CAD build for the part. Positions are in the model's coordinates, mm. A direction names the side the tool comes from. Coordinates: 2 decimals unless noted, no trailing zeros. Write item = value, one per line. Start each with the question number.
```python
from build123d import *

# Parameters (mm, degrees)
SKETCH1_R           = 10.9
BOSS_EXTRUDE1_DEPTH = 10
FILLET5_R           = 1
FILLET1_R           = 1
SKETCH3_R           = 2
CUT_EXTRUDE2_DEPTH  = 8
SKETCH6_R           = 11.874719229
SKETCH6_R_2         = 5
BOSS_EXTRUDE3_DEPTH = 3


with BuildPart() as part:
    # Sketch1 → Boss-Extrude1 (new body)
    with BuildSketch(Plane.XY):
        with BuildLine():
            Line((18.000000111, 2.53629242), (18.000000111, -9))
            Line((18.000000111, -9), (-17.965840671, -9))
            Line((-17.965840671, -9), (-17.965840671, 23.5))
            ThreePointArc((-17.965840671, 23.5), (-0.099999918, 41.365840754), (17.765840836, 23.5))
            Line((17.765840836, 23.5), (18.000000111, 16.187309001))
            Line((18.000000111, 16.187309001), (18.000000111, 14.96196947))
            Line((18.000000111, 14.96196947), (18.000000111, 2.53629242))
        make_face()
        with Locations((-0.099999918, 23.5)):
            Circle(SKETCH1_R, mode=Mode.SUBTRACT)
        with BuildLine():
            Line((-4.4, 1), (-5.2, 1))
            Line((-5.2, 1), (-6, 0.2))
            Line((-6, 0.2), (-6, -3.6))
            ThreePointArc((-6, -3.6), (-5.882842712, -3.882842712), (-5.6, -4))
            Line((-5.6, -4), (5.6, -4))
            ThreePointArc((5.6, -4), (5.882842712, -3.882842712), (6, -3.6))
            Line((6, -3.6), (6, 0.2))
            Line((6, 0.2), (5.2, 1))
            Line((5.2, 1), (4.4, 1))
            Line((4.4, 1), (4.4, 2))
            Line((4.4, 2), (5.2, 2))
            Line((5.2, 2), (6, 2.8))
            Line((6, 2.8), (6, 3.6))
            ThreePointArc((6, 3.6), (5.882842712, 3.882842712), (5.6, 4))
            Line((5.6, 4), (-5.6, 4))
            ThreePointArc((-5.6, 4), (-5.882842712, 3.882842712), (-6, 3.6))
            Line((-6, 3.6), (-6, 2.8))
            Line((-6, 2.8), (-5.2, 2))
            Line((-5.2, 2), (-4.4, 2))
            Line((-4.4, 2), (-4.4, 1))
        make_face(mode=Mode.SUBTRACT)
    extrude(amount=-BOSS_EXTRUDE1_DEPTH)

    # Fillet5
    fillet5_edges = [part.edges().sort_by_distance(p)[0] for p in [
        (18.000000111, -9, -5),
        (-17.965840671, -9, -5),
        (0.01707972, -9, -10),
        (0.01707972, -9, 0),
    ]]
    fillet(fillet5_edges, radius=FILLET5_R)

    # Fillet1
    # the kernel refuses this fillet: 1 mm, written as the material it adds along each edge
    with BuildSketch(Plane(origin=(17.765840836, 23.5, 0), x_dir=(0.032004541259538756, -0.9994877234557543, 0), z_dir=(0, 0, -1))) as fillet1_piece_1:
        with BuildLine():
            CenterArc((0.015788393, -1), FILLET1_R, 90, 1.784765128)
            ThreePointArc((-0.015356597, -0.000485123), (-0.007678246, -0.000244212), (0, 0))
            Line((0, 0), (0.015788393, 0))
        make_face()
    extrude(amount=10)
    # the kernel refuses this fillet: 1 mm, written as the material it takes off along each edge
    with BuildSketch(Plane(origin=(-17.965840671, -10.5, -10), x_dir=(1, 0, 0), z_dir=(0, 1, 0)), Plane(origin=(-17.965840671, -10.5, 0), x_dir=(0, 0, -1), z_dir=(0, 1, 0))) as fillet1_2_piece_1:
        with BuildLine():
            CenterArc((FILLET1_R, -FILLET1_R), FILLET1_R, 90, 90)
            Line((0, -FILLET1_R), (0, 0))
            Line((0, 0), (FILLET1_R, 0))
        make_face()
    extrude(amount=34, mode=Mode.SUBTRACT)
    with BuildSketch(Plane(origin=(-0.099999918, 23.5, -10), x_dir=(-1, 0, 0), z_dir=(0, -1, 0))) as fillet1_2_piece_2:
        with BuildLine():
            CenterArc((17.865840754 - FILLET1_R, -FILLET1_R), FILLET1_R, 0, 90)
            Line((17.865840754, -FILLET1_R), (17.865840754, 0))
            Line((17.865840754, 0), (17.865840754 - FILLET1_R, 0))
        make_face()
    revolve(axis=Axis((-0.099999918, 23.5, -10), (0, 0, -1)), revolution_arc=179.950726799, mode=Mode.SUBTRACT)
    with BuildSketch(Plane(origin=(-0.099999918, 23.5, 0), x_dir=(-1, 0, 0), z_dir=(0, -1, 0))) as fillet1_2_piece_3:
        with BuildLine():
            CenterArc((17.865840754 - FILLET1_R, FILLET1_R), FILLET1_R, 270, 90)
            Line((17.865840754 - FILLET1_R, 0), (17.865840754, 0))
            Line((17.865840754, 0), (17.865840754, FILLET1_R))
        make_face()
    revolve(axis=Axis((-0.099999918, 23.5, 0), (0, 0, -1)), revolution_arc=179.950726799, mode=Mode.SUBTRACT)
    with BuildSketch(Plane(origin=(18.76583386, 23.516224236, 0), x_dir=(0.8198872609406254, -0.5725250032507568, 0), z_dir=(0.5725250032507568, 0.8198872609406254, 0))) as fillet1_2_piece_4:
        with BuildLine():
            CenterArc((1 + FILLET1_R, FILLET1_R), FILLET1_R, 180, 90)
            Line((1, FILLET1_R), (1, 0))
            Line((1, 0), (1 + FILLET1_R, 0))
        make_face()
    revolve(axis=Axis((18.76583386, 23.516224236, 0), (0, 0, -1)), revolution_arc=145.024236532, mode=Mode.SUBTRACT)
    with BuildSketch(Plane(origin=(18.76583386, 23.516224236, -10), x_dir=(0.8198872609406254, -0.5725250032507568, 0), z_dir=(0.5725250032507568, 0.8198872609406254, 0))) as fillet1_2_piece_5:
        with BuildLine():
            CenterArc((1 + FILLET1_R, -FILLET1_R), FILLET1_R, 90, 90)
            Line((1, -FILLET1_R), (1, 0))
            Line((1, 0), (1 + FILLET1_R, 0))
        make_face()
    revolve(axis=Axis((18.76583386, 23.516224236, -10), (0, 0, -1)), revolution_arc=145.024236532, mode=Mode.SUBTRACT)

    # Sketch3 → Cut-Extrude2 (cut)
    with BuildSketch(Plane.XZ.offset(9)):
        with Locations((0, -4)):
            Circle(SKETCH3_R)
    extrude(amount=-CUT_EXTRUDE2_DEPTH, mode=Mode.SUBTRACT)

    # Sketch6 → Boss-Extrude3 (add)
    with BuildSketch(Plane.XY):
        with Locations((-0.099999918, 23.5)):
            Circle(SKETCH6_R)
        with Locations((-0.099999918, 23.5)):
            Circle(SKETCH6_R_2, mode=Mode.SUBTRACT)
    extrude(amount=-BOSS_EXTRUDE3_DEPTH)


solid = part.part
```
1. Probe L1, parallel to Y at x = -0.1, z = -1.35; L2, parallel to X at y = -2, z = -1; L3, parallel to Y at x = -2, z = -5.25. List the from-to ranges inside material, lowest first.
2. 3-axis set-ups, long thin cutter, end or side, ignore diameter. For faces 4 (the cylindrical face through (-8.75, 16.87, -6.45)), 5 (the flat face through (0, 4, -5)), 6 (the flat face through (0, 10, -10)): which of +Z, -Z, +X, -X, +Y, -Y reach the whole face in a straight line?
3. Mould opens along Y. For faces 1 (the cylindrical face through (-0.5, 41.36, -4.94)), 2 (the flat face through (4.4, 1.5, -4.9)), 3 (the cylindrical face through (-17.67, 7.17, -9.71)) say: released by +Y, released by -Y, zero draft, split by the parting line, or undercut.
4. Flat gauge pins, fed straight in: pin 1 (2 mm diameter, centred on y = 24.5, z = -5, fed in from +X); pin 2 (0.6 mm diameter, centred on x = 4.5, z = -7, fed in from +Y); pin 3 (2 mm diameter, centred on y = 32.5, z = -6, fed in from +X). Where does each tip first touch, or does it go through?
5. Slice it at B-B (z = -8.25). Give the number of separate pieces and of enclosed holes in the cut face, plus the area to 3 significant figures.
Calculated:
q1.L1 = -9 to -4, 4 to 18.5, 28.5 to 41.37
q1.L2 = -17.97 to -6, 6 to 18
q1.L3 = -9 to -4, 4 to 12.77, 34.23 to 41.26
q2.face_4 = -Z
q2.face_5 = +Z, -Z
q2.face_6 = -Z, +X, -X, +Y, -Y
q3.face_1 = released by +Y
q3.face_2 = undercut
q3.face_3 = zero draft
q4.pin_1 = 17.77
q4.pin_2 = 40.84
q4.pin_3 = 15.87
q5.separate_pieces = 1
q5.enclosed_holes = 2
q5.area = 1,200 mm²
